```python
from build123d import *

# Parameters (mm, degrees)
F0_W     = 90.427961
F0_H     = 118.848171
F0_R     = 1.342773
F0_R_2   = 1.5
F1_DEPTH = 25
F2_R     = 1.5
F3_DEPTH = 25


with BuildPart() as f1:
    # F0 (on Front) → F1 (new body)
    with BuildSketch(Plane.XZ):
        with Locations((13.190647, -50.225)):
            Rectangle(F0_W, F0_H)
        with Locations((45, -90.556594)):
            Circle(F0_R, mode=Mode.SUBTRACT)
        with Locations((-25, -13.556594)):
            Circle(F0_R_2, mode=Mode.SUBTRACT)
        with Locations((0, -3.556594)):
            Circle(F0_R_2, mode=Mode.SUBTRACT)
        with Locations((24.3112, -45.556594)):
            Circle(F0_R_2, mode=Mode.SUBTRACT)
        with Locations((25, -13.556594)):
            Circle(F0_R_2, mode=Mode.SUBTRACT)
    extrude(amount=F1_DEPTH)

    # F2 (on face) → F3 (cut)
    with BuildSketch(Plane.XZ.offset(25)):
        with Locations((0, -42.056594)):
            Circle(F2_R)
        with Locations((0, -72.056594)):
            Circle(F2_R)
    extrude(amount=-F3_DEPTH, mode=Mode.SUBTRACT)


solid = f1.part
```
Here's how the part is built. I have some questions about the finished solid (model axes, mm). Coordinates: 2 decimals unless noted, no trailing zeros. Order: outer loops, then holes, each group sorted by start corner. A loop starts at its lowest first (then second) coordinate and runs counter-clockwise, first axis right, second up. Notation, with made-up numbers: M -1,88 L 44,88 A10 ccw 44,94 Z; hole C 89.5,-36 d11. An arc over 180 degrees is marked long. Answer as a JSON object with one key per item and string values. Group by question number.
(1) For pin 1 (2.5 mm diameter, centred on x = 0, z = -72.06, fed in from +Y), with a flat end and sliding along its axis, tell me the tip position at first contact or that it passes through.
(2) If we mould it in two halves opening along Z, with no side actions, what happens to faces 1 (the face through (13, -25, -49)), 2 (the face through (13, -12, 9.199)), 3 (the face through (-0.33, -12.32, -5.02))? For each: released by +Z, released by -Z, zero draft, split by the parting line, or undercut.
(3) I need wall thicknesses on probe 1 along Z at (x, y) = (0, -19.75); probe 2 along X at (y, z) = (-4.75, -12.5); probe 3 along Z at (x, y) = (-25, -8.25). Which ranges of each line are inside material? Lowest first, please.
(4) Suppose I cut it at B-B, the plane x = 45. Please give me the cut outline in (y, z), then the cut area to 3 significant figures.
(5) Suppose I cut it at A-A, the plane x = -25. Please give me the cut outline in (y, z).
Values found:
{
 "1": {"pin 1": "passes through"},
 "2": {"face 1": "zero draft", "face 2": "released by +Z", "face 3": "undercut"},
 "3": {"probe 1": "z = -109.65 to -73.56, -70.56 to -43.56, -40.56 to -5.06, -2.06 to 9.2", "probe 2": "x = -32.02 to -26.06, -23.94 to 23.94, 26.06 to 58.4", "probe 3": "z = -109.65 to -15.06, -12.06 to 9.2"},
 "4": {"outline": "M -25,-109.65 L 0,-109.65 L 0,-91.9 L -25,-91.9 Z; M -25,-89.21 L 0,-89.21 L 0,9.2 L -25,9.2 Z", "area": "2,900 mm^2"},
 "5": {"outline": "M -25,-109.65 L 0,-109.65 L 0,-15.06 L -25,-15.06 Z; M -25,-12.06 L 0,-12.06 L 0,9.2 L -25,9.2 Z"}
}
